from build123d import *

# Parameters (mm, degrees)
SKETCH1_W           = 36.83
SKETCH1_H           = 20.32
BOSS_EXTRUDE1_DEPTH = 18.796
FILLET1_R           = 3.175
BOSS_EXTRUDE2_DEPTH = 25.908
BOSS_EXTRUDE3_DEPTH = 8.382
SKETCH4_R           = 1.016
CUT_EXTRUDE1_DEPTH  = 19.796


with BuildPart() as part:
    # Sketch1 → Boss-Extrude1 (new body)
    with BuildSketch(Plane.XY):
        with Locations((18.415, 0)):
            Rectangle(SKETCH1_W, SKETCH1_H)
    extrude(amount=BOSS_EXTRUDE1_DEPTH)

    # Fillet1
    fillet1_edges = [part.edges().sort_by_distance(p)[0] for p in [
        (36.83, 10.16, 9.398),
        (36.83, -10.16, 9.398),
    ]]
    fillet(fillet1_edges, radius=FILLET1_R)

    # Sketch2 → Boss-Extrude2 (add)
    with BuildSketch(Plane.ZY):
        with BuildLine():
            ThreePointArc((3.96514897, 10.16), (1.809887501, 8.860648824), (0, 7.112))
            Line((0, 7.112), (0, -7.112))
            ThreePointArc((0, -7.112), (1.809887501, -8.860648824), (3.96514897, -10.16))
            Line((3.96514897, -10.16), (13.276942782, -10.16))
            ThreePointArc((13.276942782, -10.16), (15.61217315, -8.719352926), (17.526, -6.753130241))
            Line((17.526, -6.753130241), (17.526, 6.753130241))
            ThreePointArc((17.526, 6.753130241), (15.61217315, 8.719352926), (13.276942782, 10.16))
            Line((13.276942782, 10.16), (3.96514897, 10.16))
        make_face()
    extrude(amount=BOSS_EXTRUDE2_DEPTH)

    # Sketch3 → Boss-Extrude3 (add)
    with BuildSketch(Plane.XY.offset(18.796)):
        with BuildLine():
            Line((24.267261803, 2.273434446), (23.149675051, -1.177980315))
            ThreePointArc((23.149675051, -1.177980315), (24.617532764, -2.416473676), (26.532738197, -2.273434446))
            Line((26.532738197, -2.273434446), (27.650324949, 1.177980315))
            ThreePointArc((27.650324949, 1.177980315), (26.182467236, 2.416473676), (24.267261803, 2.273434446))
        make_face()
    extrude(amount=BOSS_EXTRUDE3_DEPTH)

    # Sketch4 → Cut-Extrude1 (cut, through all)
    with BuildSketch(Plane.XY.offset(18.796)):
        with Locations((3.456249115, 8.597457961)):
            Circle(SKETCH4_R)
        with Locations((3.456249115, -8.597457961)):
            Circle(SKETCH4_R)
    extrude(amount=-CUT_EXTRUDE1_DEPTH, mode=Mode.SUBTRACT)


solid = part.part
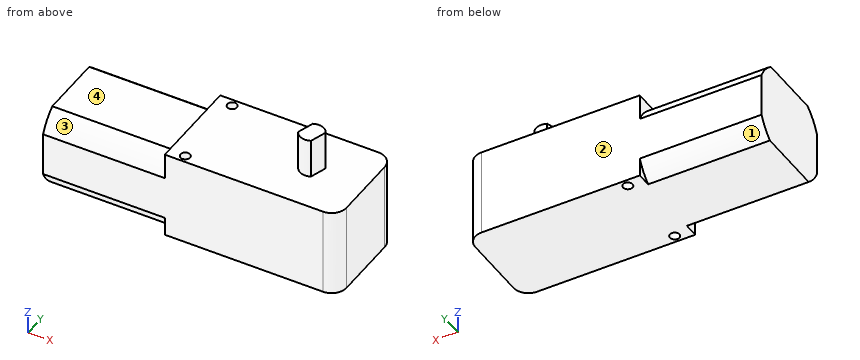
CAD build for the part. Positions are in the model's coordinates, mm. Face numbers are marked on the shaded views. A direction names the side the tool comes from. Round coordinates to 2 decimals unless told otherwise and drop trailing zeros. Order: outer loops, then holes, each group sorted by start corner. A loop starts at its lowest first (then second) coordinate and runs counter-clockwise, first axis right, second up. Notation, with made-up numbers: (85, -2.5) -> (123, -2.5) arc R20 ccw to (123, 13.5) -> close; hole circle Ø2 at (67, 26). An arc over 180 degrees is marked (long way). Write item = value, one per line. Start each with the question number.
(1) Cut at D-D, the plane z = 20.5. List the corners of the cut face in (x, y).
(2) Which spindle directions (+Z, -Z, +X, -X, +Y, -Y) get a long thin tool onto all of the face, cutting with end or side? Do the marked faces 1, 2, 3 and 4. Say none if no direction does.
(3) Probe line 1 (Z direction, x = 30.5, y = 6); line 2 (Z direction, x = -3, y = -5); line 3 (Y direction, x = 25, z = 19.25). List the from-to ranges inside material, lowest first. Write a range as [from, to].
(4) Pin check, flat tips, straight feed: P1, Ø8, axis at x = -12.5, y = -6, coming from the +Z side; P2, Ø6, axis at x = 16, y = -0.5, coming from the +Z side. Stop position of each tip, or through.
(5) Cut at C-C, the plane x = -15. List the corners of the cut face in (y, z), then the cut area to 3 significant figures.
(6) Cut at B-B, the plane y = 5.5. List the corners of the cut face in (x, z), then the cut area to 3 significant figures.
(7) Cut at A-A, the plane z = 15. List the corners of the cut face in (x, y) (3 decimals).
Model answer:
q1.outline = (23.15, -1.18) arc R2.54 ccw to (26.53, -2.27) -> (27.65, 1.18) arc R2.54 ccw to (24.27, 2.27) -> close
q2.face_1 = -Z, -X, +Y
q2.face_2 = +Z, -Z, +X, -X, +Y
q2.face_3 = +Z, -X, -Y
q2.face_4 = +Z, -X, +Y, -Y
q3.line_1 = [0, 18.8]
q3.line_2 = [0, 17.53]
q3.line_3 = [-2.51, 2.51]
q4.P1 = 17.53
q4.P2 = 18.8
q5.outline = (-10.16, 3.97) arc R11.18 ccw to (-7.11, 0) -> (7.11, 0) arc R11.18 ccw to (10.16, 3.97) -> (10.16, 13.28) arc R11.18 ccw to (6.75, 17.53) -> (-6.75, 17.53) arc R11.18 ccw to (-10.16, 13.28) -> close
q5.area = 334 mm2
q6.outline = (-25.91, 0) -> (36.83, 0) -> (36.83, 18.8) -> (0, 18.8) -> (0, 17.53) -> (-25.91, 17.53) -> close
q6.area = 1,150 mm2
q7.outline = (-25.908, -9.177) -> (0, -9.177) -> (0, -10.16) -> (33.655, -10.16) arc R3.175 ccw to (36.83, -6.985) -> (36.83, 6.985) arc R3.175 ccw to (33.655, 10.16) -> (0, 10.16) -> (0, 9.177) -> (-25.908, 9.177) -> close; hole circle Ø2.032 at (3.456, -8.597); hole circle Ø2.032 at (3.456, 8.597)
